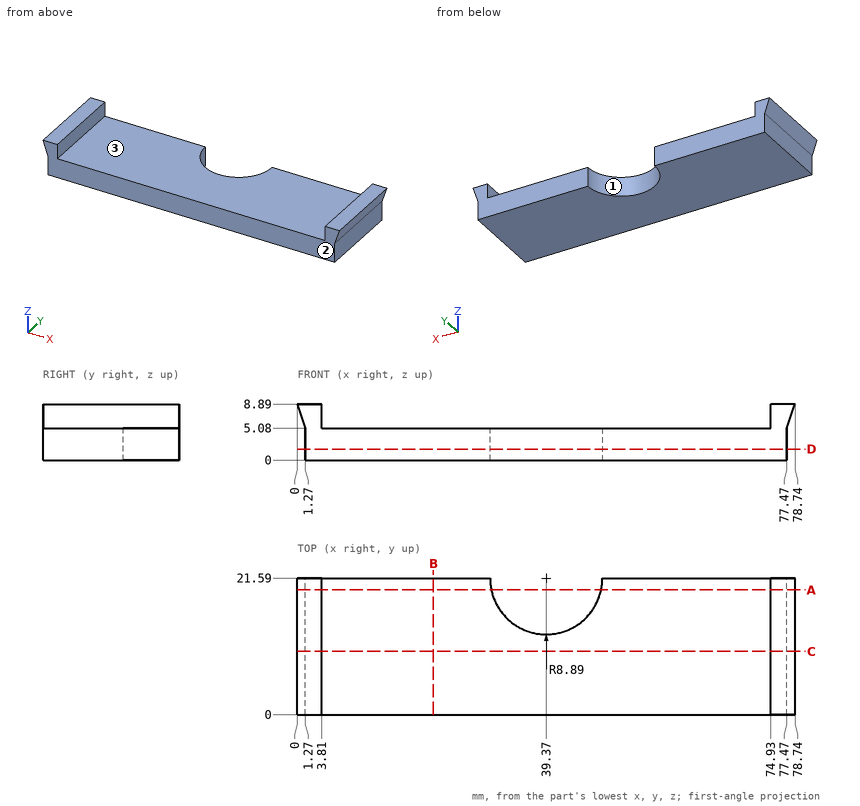
Job drawing, mm, ordinate dimensions from the low corner. One solid piece. Round coordinates to 2 decimals unless told otherwise and drop trailing zeros. Write each loop counter-clockwise with the first axis right and the second up, starting at its lowest first coordinate (ties: lowest second). Pieces come first, ordered by that corner, then holes.
1) Mould opens along X. For the marked faces 1, 2 and 3 say: +X half, -X half, draft (parallel to the pull), parting line (faces both ways), or undercut.
2) Band-saw the part on C-C, the plane y = 10. List the corners of the cut face in (x, z).
3) Drill centre lines: probe 1 along X at (y, z) = (11, 1.75); probe 2 along Z at (x, y) = (21.5, 17.5); probe 3 along X at (y, z) = (18.75, 3.5). Where is each one in solid material? Low to high.
4) Pin check, flat tips, straight feed: pin 1 (1.5 mm diameter, centred on y = 10.5, z = 3, fed in from +X); pin 2 (3 mm diameter, centred on y = 15.5, z = 7, fed in from -X); pin 3 (1.5 mm diameter, centred on y = 9, z = 2, fed in from -X). Stop position of each tip, or through.
5) Band-saw the part on D-D, the plane z = 1.75. List the corners of the cut face in (x, y).
6) Band-saw the part on A-A, the plane y = 19.75. List the corners of the cut face in (x, z), and give its area (3 significant figures).
7) Band-saw the part on B-B, the plane x = 21.5. List the corners of the cut face in (y, z), and give its area (3 significant figures).
Ans:
1. face 1: undercut
1. face 2: draft
1. face 3: undercut
2. outline: (0, 8.89) - (1.27, 5.08) - (1.27, 0) - (77.47, 0) - (77.47, 5.08) - (78.74, 8.89) - (74.93, 8.89) - (74.93, 5.08) - (3.81, 5.08) - (3.81, 8.89) - close
3. probe 1: x = 1.27 to 77.47
3. probe 2: z = 0 to 5.08
3. probe 3: x = 1.27 to 30.95, 47.79 to 77.47
4. pin 1: stops at x = 77.47
4. pin 2: stops at x = 0.13
4. pin 3: stops at x = 1.27
5. outline: (1.27, 0) - (77.47, 0) - (77.47, 21.59) - (48.26, 21.59) arc R8.89 cw to (30.48, 21.59) - (1.27, 21.59) - close
6. outline: (0, 8.89) - (1.27, 5.08) - (1.27, 0) - (30.67, 0) - (30.67, 5.08) - (3.81, 5.08) - (3.81, 8.89) - close; (48.07, 0) - (77.47, 0) - (77.47, 5.08) - (78.74, 8.89) - (74.93, 8.89) - (74.93, 5.08) - (48.07, 5.08) - close
6. area: 323 mm2
7. outline: (0, 0) - (21.59, 0) - (21.59, 5.08) - (0, 5.08) - close
7. area: 110 mm2
